Here's how the part is built. I have some questions about the finished solid (model axes, mm). A direction names the side the tool comes from. Round coordinates to 2 decimals unless told otherwise and drop trailing zeros. Loops run counter-clockwise (first coordinate to the right, second up) from the corner with the lowest first, then second, coordinate; pieces in that order, holes last. Notation, with made-up numbers: M 85,31.5 L 144,31.5 A15 ccw 144,39.5 Z; hole C 18,39.5 d7. An arc over 180 degrees is marked long. Use a Markdown table: item, result.
```python
from build123d import *

# Parameters (mm, degrees)
SKETCH1_W           = 26
SKETCH1_H           = 25.1
BOSS_EXTRUDE1_DEPTH = 2.05
CUT_EXTRUDE1_DEPTH  = 19.185296258
SKETCH3_R           = 2.5
BOSS_EXTRUDE2_DEPTH = 6
SKETCH4_R           = 7
BOSS_EXTRUDE3_DEPTH = 1
SKETCH5_R           = 1.4
CUT_EXTRUDE2_DEPTH  = 9.05


with BuildPart() as part:
    # Sketch1 → Boss-Extrude1 (new body)
    with BuildSketch(Plane.XY):
        Rectangle(SKETCH1_W, SKETCH1_H)
    extrude(amount=BOSS_EXTRUDE1_DEPTH)

    # Sketch2 → Cut-Extrude1 (cut, through all)
    with BuildSketch(Plane.XY.offset(2.05)):
        with BuildLine():
            Line((-8.46, -5.25), (-8.46, 6.75))
            ThreePointArc((-8.46, 6.75), (-10, 8.29), (-11.54, 6.75))
            Line((-11.54, 6.75), (-11.54, -5.25))
            ThreePointArc((-11.54, -5.25), (-10, -6.79), (-8.46, -5.25))
        make_face()
        with BuildLine():
            ThreePointArc((-2.002069244, -2.286766992), (-1.773484699, 2.732003629), (2.438049628, 5.471216664))
            Line((2.438049628, 5.471216664), (2.438049628, 6.475663038))
            ThreePointArc((2.438049628, 6.475663038), (-2.615725538, 3.273167683), (-2.91153638, -2.702542808))
            Line((-2.91153638, -2.702542808), (-2.002069244, -2.286766992))
        make_face()
        with BuildLine():
            Line((3.517695015, 6.479351192), (3.438049628, 5.482527932))
            ThreePointArc((3.438049628, 5.482527932), (7.742278908, 2.785819585), (8.002069244, -2.286766992))
            Line((8.002069244, -2.286766992), (8.91153638, -2.702542808))
            ThreePointArc((8.91153638, -2.702542808), (8.604511436, 3.292332237), (3.517695015, 6.479351192))
        make_face()
        with BuildLine():
            ThreePointArc((7.505336244, -3.1546704), (3, -5.5), (-1.505336244, -3.1546704))
            Line((-1.505336244, -3.1546704), (-2.324488288, -3.728246836))
            ThreePointArc((-2.324488288, -3.728246836), (3, -6.5), (8.324488288, -3.728246836))
            Line((8.324488288, -3.728246836), (7.505336244, -3.1546704))
        make_face()
    extrude(amount=-CUT_EXTRUDE1_DEPTH, mode=Mode.SUBTRACT)

    # Sketch3 → Boss-Extrude2 (add)
    with BuildSketch(Plane.XY.offset(2.05)):
        with Locations(Location((-4.071067812, 7.071067812, 0), (0, 0, 180))):
            Circle(SKETCH3_R)
        with Locations(Location((10.071067812, 7.071067812, 0), (0, 0, 180))):
            Circle(SKETCH3_R)
        with Locations(Location((10.071067812, -7.071067812, 0), (0, 0, 180))):
            Circle(SKETCH3_R)
        with Locations(Location((-4.071067812, -7.071067812, 0), (0, 0, 180))):
            Circle(SKETCH3_R)
    extrude(amount=BOSS_EXTRUDE2_DEPTH)

    # Sketch4 → Boss-Extrude3 (add)
    with BuildSketch(Plane.XY.offset(8.05)):
        with BuildLine():
            Line((-4.071067812, 9.571067812), (10.071067812, 9.571067812))
            ThreePointArc((10.071067812, 9.571067812), (11.838834765, 8.838834765), (12.571067812, 7.071067812))
            Line((12.571067812, 7.071067812), (12.571067812, -7.071067812))
            ThreePointArc((12.571067812, -7.071067812), (11.838834765, -8.838834765), (10.071067812, -9.571067812))
            Line((10.071067812, -9.571067812), (-4.071067812, -9.571067812))
            ThreePointArc((-4.071067812, -9.571067812), (-5.838834765, -8.838834765), (-6.571067812, -7.071067812))
            Line((-6.571067812, -7.071067812), (-6.571067812, 7.071067812))
            ThreePointArc((-6.571067812, 7.071067812), (-5.838834765, 8.838834765), (-4.071067812, 9.571067812))
        make_face()
        with Locations((3, 0)):
            Circle(SKETCH4_R, mode=Mode.SUBTRACT)
    extrude(amount=BOSS_EXTRUDE3_DEPTH)

    # Sketch5 → Cut-Extrude2 (cut)
    with BuildSketch(Plane.XY.offset(9.05)):
        with Locations((-4.071067812, -7.071067812)):
            Circle(SKETCH5_R)
        with Locations((-4.071067812, 7.071067812)):
            Circle(SKETCH5_R)
        with Locations((10.071067812, 7.071067812)):
            Circle(SKETCH5_R)
        with Locations((10.071067812, -7.071067812)):
            Circle(SKETCH5_R)
    extrude(amount=-CUT_EXTRUDE2_DEPTH, mode=Mode.SUBTRACT)


solid = part.part
```
Q1. Will these pins go through, and if not, where does the flat tip stop? P1, Ø11, axis at x = 3, y = 0, coming from the -Z side; P2, Ø2.5, axis at x = -4.07, y = -7.07, coming from the -Z side; P3, Ø0.5, axis at x = 3.5, z = 8.5, coming from the -Y side; P4, Ø1.1, axis at x = 5.5, z = 8.5, coming from the +Y side.
Return value:
| item | result |
|---|---|
| P1 | stops at z = 0 |
| P2 | passes through |
| P3 | stops at y = -9.57 |
| P4 | stops at y = 9.57 |
Q2. Imagine slicing it at A-A, the plane z = 3.25. Please give me the cut outline in (x, y), then the cut area to 3 significant figures.
Return value:
| item | result |
|---|---|
| outline | C -4.07,-7.07 d5; C -4.07,7.07 d5; C 10.07,-7.07 d5; C 10.07,7.07 d5; hole C -4.07,-7.07 d2.8; hole C -4.07,7.07 d2.8; hole C 10.07,-7.07 d2.8; hole C 10.07,7.07 d2.8 |
| area | 53.9 mm^2 |
Q3. For faces 1 (the flat face through (7, 6, 8.05)), 2 (the flat face through (-11.54, 1, 1)), 3 (the flat face through (3.1, -9.571, 8.5)), 4 (the flat face through (-6.571, -0.1, 8.5)), which set-ups out of +Z, -Z, +X, -X, +Y, -Y let a thin tool reach every point of the face, with its end or its side?
Return value:
| item | result |
|---|---|
| face 1 | none |
| face 2 | +Z, -Z |
| face 3 | +Z, +X, -X, -Y |
| face 4 | +Z, -X, +Y, -Y |
Q4. Imagine slicing it at D-D, the plane z = 1.25. Give the number of separate pieces and of enclosed holes in the cut face, then the cut area to 3 significant figures.
Return value:
| item | result |
|---|---|
| separate pieces | 1 |
| enclosed holes | 8 |
| area | 549 mm^2 |
Q5. Imagine slicing it at C-C, the plane x = 3. Please give me the cut outline in (y, z).
Return value:
| item | result |
|---|---|
| outline | M -12.55,0 L -6.5,0 L -6.5,2.05 L -12.55,2.05 Z; M -9.57,8.05 L -7,8.05 L -7,9.05 L -9.57,9.05 Z; M -5.5,0 L 12.55,0 L 12.55,2.05 L -5.5,2.05 Z; M 7,8.05 L 9.57,8.05 L 9.57,9.05 L 7,9.05 Z |
Q6. Imagine slicing it at B-B, the plane y = 7.5. Please give me the cut outline in (x, z), then the cut area to 3 significant figures.
Return value:
| item | result |
|---|---|
| outline | M -13,0 L -11.35,0 L -11.35,2.05 L -13,2.05 Z; M -8.65,0 L -5.4,0 L -5.4,9.05 L -6.53,9.05 L -6.53,2.05 L -8.65,2.05 Z; M -2.74,0 L 8.74,0 L 8.74,9.05 L -2.74,9.05 Z; M 11.4,0 L 13,0 L 13,2.05 L 12.53,2.05 L 12.53,9.05 L 11.4,9.05 Z; hole M -1.61,2.05 L 7.61,2.05 L 7.61,8.05 L -1.61,8.05 Z |
| area | 77.7 mm^2 |
Q7. I need wall thicknesses on line 1 (X direction, y = -7.5, z = 0.5); line 2 (X direction, y = 1.5, z = 1); line 3 (Y direction, x = 7, z = 0.5). Which ranges of each line are inside material? Lowest first, please. Write a range as from..to.
Return value:
| item | result |
|---|---|
| line 1 | x = -13..-5.4, -2.74..8.74, 11.4..13 |
| line 2 | x = -13..-11.54, -8.46..-3.32, -2.29..8.29, 9.32..13 |
| line 3 | y = -12.55..-5.12, -3.77..3.77, 5.12..12.55 |
Q8. We'd pull the mould along X, two halves only. Please class faces 5 (the flat face through (7, 7, 9.05)), 6 (the flat face through (3.48, 5.99, 1.04)), 7 (the flat face through (13, 0, 1)), 8 (the cylindrical face through (3.1, -5.5, 1)): pulls with the +X half, pulls with the -X half, needs draft (parallel to the pull), parting line crosses it, or undercut.
Return value:
| item | result |
|---|---|
| face 5 | needs draft |
| face 6 | undercut |
| face 7 | pulls with the +X half |
| face 8 | undercut |
